Can you work these out from the model? Positions are in its coordinate system, mm. A direction names the side the tool comes from. Round coordinates to 2 decimals unless told otherwise and drop trailing zeros. Write each loop counter-clockwise with the first axis right and the second up, starting at its lowest first coordinate (ties: lowest second). Pieces come first, ordered by that corner, then holes. Notation, with made-up numbers: (22.5, 0.5) - (39.5, 0.5) arc R29 cw to (39.5, 28.5) - close; hole circle Ø8 at (72.5, 82.25). An arc over 180 degrees is marked (long way). One line per item, written item: value. Start each with the question number.
(1) Thinking about a two-plate mould opening in Y: for faces 1 (the face through (-12.229, -63.904, -19.968)), 2 (the face through (11.2, -63.9, -20.6)), 3 (the face through (10, -97.58, -24)), 4 (the face through (-24.11, -84.88, -8.12)), which applies, +Y half, -Y half, draft (parallel to the pull), parting line (faces both ways), or undercut?
(2) On a 3-axis mill with a long thin cutter (end or side, diameter ignored), from which of +Z, -Z, +X, -X, +Y, -Y can I reach the whole of each face in a straight line? I mean faces 5 (the face through (-23.4, -63.9, 0.6)), 6 (the face through (0.6, -63.9, 23.4)), 7 (the face through (10.5, -65.93, 18.35)). Say none if no direction works.
(3) I want a section at A-A on y = -31.5. List the corners of the cut face in (x, z) for me.
(4) If I drill on L1, parallel to X at y = -23.5, z = 0; L2, parallel to X at y = -27, z = 0 (3 decimals); L3, parallel to X at y = -65, z = -9.5, over which ranges is the centre line in solid material (lowest first)? Write a range as from..to.
(5) I'm going to push flat-ended pins straight in: pin 1 Ø12 at (y, z) = (-51.5, -10.5) entering from -X; pin 2 Ø12 at (y, z) = (-78, -4) entering from +X; pin 3 Ø13.5 at (x, z) = (4.5, 2) entering from +Y; pin 4 Ø2 at (x, y) = (-2.5, -87) entering from -Z. Where does each tip first touch, or does it pass through?
from build123d import *

# Parameters (mm, degrees)
CIRPATTERN1_COUNT = 12


with BuildPart() as part:
    # Sketch1 → Revolve1 (revolve)
    with BuildSketch(Plane.XY, mode=Mode.PRIVATE) as revolve1_sk:
        Polygon((19.05, -29.351053449), (19.05, -60.847053449), (25.2857, -60.847053449), (25.2857, -36.971053449), (22.225, -36.971053449), (22.225, -33.161053449), (25.2857, -33.161053449), (25.2857, -17.794053449), (20.447, -17.794053449), (19.05, -19.191053449), (19.05, -25.541053449), (22.225, -25.541053449), (22.225, -29.351053449), align=None)
        Polygon((25.2857, -84.879763523), (26.9875, -84.879763523), (26.9875, -97.579763523), (25.7175, -97.579763523), (15.875, -60.847053449), (19.05, -60.847053449), (25.2857, -60.847053449), align=None)
    revolve(revolve1_sk.sketch.rotate(Axis((0, 0, 0), (0, 1, 0)), 90), axis=Axis((0, 0, 0), (0, 1, 0)))

    # Sketch3 → #10-32 Tapped Hole1 (revolve, cut)
    with BuildSketch(Plane(origin=(0, -65.829763523, -25.2857), x_dir=(0, 1, 0), z_dir=(1, 0, 0))):
        Polygon((0, 0), (0, 4.166057072), (2.0193, 3.81), (2.0193, 0), align=None)
    f_10_32_tapped_hole1 = revolve(axis=Axis((0, -65.829763523, -31.6357), (0, 0, 1)), mode=Mode.SUBTRACT)

    # CirPattern1: #10-32 Tapped Hole1 ×12 about axis
    cirpattern1_axis = Axis((0, 0, 0), (0, -1, 0))
    for i in range(1, CIRPATTERN1_COUNT):
        add(f_10_32_tapped_hole1.rotate(cirpattern1_axis, i * 360 / CIRPATTERN1_COUNT), mode=Mode.SUBTRACT)


solid = part.part
Established:
1. face 1: undercut
1. face 2: undercut
1. face 3: -Y half
1. face 4: +Y half
2. face 5: -X
2. face 6: +Z
2. face 7: none
3. outline: circle Ø50.57 at (0, 0); hole circle Ø38.1 at (0, 0)
4. L1: -25.29..-19.05, 19.05..25.29
4. L2: -25.286..-22.225, 22.225..25.286
4. L3: -23.43..-20.14, -19.23..-14.08, 14.08..19.23, 20.14..23.43
5. pin 1: x = -24.88
5. pin 2: x = 25.29
5. pin 3: through
5. pin 4: z = -26.95
